```python
from build123d import *

# Parameters (mm, degrees)
F1_DEPTH      = 3
F1_DEPTH_BACK = 3
F0_R          = 15
F2_DEPTH      = 3
F3_DEPTH      = 3


with BuildPart() as f1:
    # F0 (on Right) → F1 (new body, two sides)
    with BuildSketch(Plane.YZ) as f1_sk:
        with BuildLine():
            ThreePointArc((-70, 30), (-48.786797, 21.213203), (-40, 0))
            ThreePointArc((-40, 0), (-48.786797, -21.213203), (-70, -30))
            Line((-70, -30), (0, -30))
            ThreePointArc((0, -30), (-30, 0), (0, 30))
            Line((0, 30), (-70, 30))
        make_face()
    extrude(amount=F1_DEPTH)
    extrude(f1_sk.sketch, amount=-F1_DEPTH_BACK)

    # F0 (on Right) → F2 (join)
    with BuildSketch(Plane.YZ):
        with BuildLine():
            ThreePointArc((30, 0), (21.213203, 21.213203), (0, 30))
            ThreePointArc((0, 30), (-30, 0), (0, -30))
            ThreePointArc((0, -30), (21.213203, -21.213203), (30, 0))
        make_face()
        Circle(F0_R, mode=Mode.SUBTRACT)
    extrude(amount=F2_DEPTH)

    # F0 (on Right) → F3 (join)
    with BuildSketch(Plane.YZ):
        with BuildLine():
            ThreePointArc((-70, -30), (-48.786797, -21.213203), (-40, 0))
            ThreePointArc((-40, 0), (-48.786797, 21.213203), (-70, 30))
            ThreePointArc((-70, 30), (-100, 0), (-70, -30))
        make_face()
        with Locations((-70, 0)):
            Circle(F0_R, mode=Mode.SUBTRACT)
    extrude(amount=-F3_DEPTH)


solid = f1.part
```
Design review of the part built by this model. Coordinates are the model's own, in mm. A direction names the side the tool comes from. Coordinates: 2 decimals unless noted, no trailing zeros. Write each loop counter-clockwise with the first axis right and the second up, starting at its lowest first coordinate (ties: lowest second). Pieces come first, ordered by that corner, then holes.
1) Add section C-C (y = -73.5). Write out the cut boundary in (x, z), plus the area to 3 significant figures.
2) Add section B-B (x = 0.9). Write out the cut boundary in (y, z), plus the area to 3 significant figures.
3) Mouldability with a two-part tool opening along Z and no side actions: class faces 4 (the flat face through (3, -21, 0)), 5 (the flat face through (0, -35, -30)), 6 (the cylindrical face through (-1.479, -84.985, 0.66)) as +Z half, -Z half, draft (parallel to the pull), parting line (faces both ways), or undercut.
4) To check wall thickness, follow L1, parallel to Z at x = -0.8, y = -69.5; L2, parallel to X at y = 21, z = 8.5; L3, parallel to Y at x = -0.05, z = 0.5. State the ranges of each line that lie inside material, in increasing order.
5) Add section A-A (z = 18). Write out the cut boundary in (x, y), plus the area to 3 significant figures.
6) Machinability: for faces 1 (the flat face through (0, -64, 14)), 2 (the flat face through (0, -35, 30)), 3 (the cylindrical face through (-1.479, -29.993, -0.66)), which of the approach directions +Z, -Z, +X, -X, +Y, -Y give a long, thin tool a straight path to every point of the face, cutting with its end or side? Answer none if there is none.
7) Insertion check: pin 1 (3 mm diameter, centred on x = 1.5, z = -14.5, fed in from +Y); pin 2 (1.5 mm diameter, centred on y = -58.5, z = 11, fed in from +X); pin 3 (1 mm diameter, centred on x = -1.5, z = -22, fed in from +Y); pin 4 (10 mm diameter, centred on y = -8, z = -2, fed in from +X). Each pin has a flat end and moves straight along its axis. Give the tip position at first contact, or say it passes through.
8) Add section D-D (z = -2.5). Write out the cut boundary in (x, y), plus the area to 3 significant figures.
Check result:
1. outline: (-3, -29.8) - (0, -29.8) - (0, -14.59) - (-3, -14.59) - close; (-3, 14.59) - (0, 14.59) - (0, 29.8) - (-3, 29.8) - close
1. area: 91.3 mm2
2. outline: (-70, -30) - (0, -30) arc R30 ccw to (30, 0) arc R30 ccw to (0, 30) - (-70, 30) arc R30 cw to (-40, 0) arc R30 cw to start; hole circle Ø30 at (0, 0)
2. area: 3,490 mm2
3. face 4: draft
3. face 5: -Z half
3. face 6: undercut
4. L1: z = -30 to -14.99, 14.99 to 30
4. L2: x = 0 to 3
4. L3: y = -100 to -84.99, -55.01 to -30
5. outline: (-3, -94) - (0, -94) - (0, -46) - (3, -46) - (3, 24) - (0, 24) - (0, -24) - (-3, -24) - close
5. area: 420 mm2
6. face 1: +X, -Y
6. face 2: +Z, +X, -X, +Y, -Y
6. face 3: -X, +Y
7. pin 1: stops at y = 27.04
7. pin 2: stops at x = 0
7. pin 3: stops at y = -19.84
7. pin 4: passes through
8. outline: (-3, -99.9) - (0, -99.9) - (0, -84.79) - (-3, -84.79) - close; (-3, -55.21) - (0, -55.21) - (0, -40.1) - (3, -40.1) - (3, -14.79) - (0, -14.79) - (0, -29.9) - (-3, -29.9) - close; (0, 14.79) - (3, 14.79) - (3, 29.9) - (0, 29.9) - close
8. area: 243 mm2
